```python
from build123d import *

# Parameters (mm, degrees)
F0_W     = 10
F0_H     = 5
F1_DEPTH = 5
F6_DEPTH = 2.8877513459


# Not quite as in the source:
# - a pattern or mirror of a feature is missing from the dataset's text; its kind, count and spacing are read off the source's solid


with BuildPart() as f1:
    # F0 (on Right) → F1 (new body, symmetric)
    with BuildSketch(Plane.YZ):
        with Locations((5, 2.5)):
            Rectangle(F0_W, F0_H)
        Polygon((10, 0), (0, 0), (5, -5), (10, -5), align=None)
    extrude(amount=F1_DEPTH, both=True)

    # F5 (on 3pt) → F6 (cut, through all)
    with BuildSketch(Plane(origin=(1.6666666667, -1.6666666667, 1.6666666667), x_dir=(0.8164965809, 0.4082482905, -0.4082482905), z_dir=(-0.5773502692, 0.5773502692, -0.5773502692))):
        Polygon((4.0824829046, 0), (-2.0412414523, -3.5355339059), (4.0824829046, -7.0710678119), align=None)
    f6 = extrude(amount=-F6_DEPTH, mode=Mode.SUBTRACT)

    # F6_copies: F6 across plane
    add(f6.mirror(Plane(origin=(0, 0, 0), x_dir=(0, 0, -1), z_dir=(-1, 0, 0))), mode=Mode.SUBTRACT)


solid = f1.part
```
For this review, take the finished solid that the model builds, in its own axes (mm). Give positions to 0.01 mm unless a question says otherwise; leave off trailing zeros. Write each loop counter-clockwise with the first axis right and the second up, starting at its lowest first coordinate (ties: lowest second). Pieces come first, ordered by that corner, then holes. Notation, with made-up numbers: M -29,89 L 29,89 A18 cw 29,103 Z; hole C -11,49.5 d4. An arc over 180 degrees is marked long. Answer as a JSON object with one key per item and string values. Group by question number.
Item 1: Consider section D-D on z = -2.25. Write out the cut boundary in (x, y).
Item 2: Consider section C-C on z = -0.25. Write out the cut boundary in (x, y).
Item 3: For pin 1 Ø1.5 at (x, z) = (-2, -2) entering from -Y, flat-tipped, find the tip position at first contact; note if it passes through.
Item 4: For probe 1 along Z at (x, y) = (-3.5, 4.25); probe 2 along Z at (x, y) = (2, 1.5); probe 3 along Y at (x, z) = (-2.5, 4), list the stretches that pass through material, from the lowest coordinate up. Write a range as [from, to].
Item 5: Consider section B-B on y = 4. Write out the cut boundary in (x, z), plus the area to 3 significant figures.
Item 6: Consider section A-A on x = -1.5. Write out the cut boundary in (y, z).
Check result:
{
 "1": {"outline": "M -5,2.25 L 5,2.25 L 5,10 L -5,10 Z"},
 "2": {"outline": "M -5,0.25 L 5,0.25 L 5,10 L -5,10 Z"},
 "3": {"pin 1": "stops at y = 1.25"},
 "4": {"probe 1": "z = [-4.25, 5]", "probe 2": "z = [-1.5, 4.5]", "probe 3": "y = [1.5, 10]"},
 "5": {"outline": "M -5,-4 L 5,-4 L 5,4 L 4,5 L -4,5 L -5,4 Z", "area": "89.0 mm^2"},
 "6": {"outline": "M 0,0 L 5,-5 L 10,-5 L 10,5 L 1.5,5 L 0,3.5 Z"}
}
